The model under review builds one solid part; all positions refer to its coordinate system, in mm. Face numbers are marked on the shaded views. A direction names the side the tool comes from. Round coordinates to 2 decimals unless told otherwise and drop trailing zeros. Write each loop counter-clockwise with the first axis right and the second up, starting at its lowest first coordinate (ties: lowest second). Pieces come first, ordered by that corner, then holes. Notation, with made-up numbers: (-11, 86) -> (33, 86) arc R22 cw to (33, 101) -> close; hole circle Ø10 at (52.5, 86.5). An arc over 180 degrees is marked (long way). Return JSON: item names as keys, results as strings. Group by question number.
1. Tool access review of the marked faces 5, 6 and 7: name each direction out of +Z, -Z, +X, -X, +Y, -Y from which nothing blocks a thin tool from reaching the whole face with its end or side.
2. Take a section at A-A, the plane x = -60. Write out the cut boundary in (y, z).
3. Clearance check with flat-ended pins moving along their axes: P1, Ø4, axis at x = -89.5, z = 44, coming from the +Y side; P2, Ø4, axis at y = -20, z = -13.5, coming from the +X side; P3, Ø8, axis at x = -8.5, y = -31.5, coming from the +Z side; P4, Ø5.5, axis at x = -83.5, y = -37, coming from the +Z side. State where each tip first meets the part, or that it passes through.
4. Take a section at D-D, the plane x = -89. Write out the cut boundary in (y, z), then the cut area to 3 significant figures.
5. Mouldability with a two-part tool opening along Z and no side actions: class the marked faces 1, 2, 3 and 4 as pulls with the +Z half, pulls with the -Z half, needs draft (parallel to the pull), parting line crosses it, or undercut.
6. Take a section at B-B, the plane y = -3.5. Write out the cut boundary in (x, z), then the cut area to 3 significant figures.
7. Take a section at C-C, the plane z = 23. Write out the cut boundary in (x, y), then the cut area to 3 significant figures.
8. For line 1 along Y through (x, z) = (-63.5, 57.5) (3 decimals); line 2 along Z through (x, y) = (-63.5, -47); line 3 along X through (y, z) = (-44, -16), list the stretches that pass through material, from the lowest coordinate up. Write a range as from..to.
from build123d import *

# Parameters (mm, degrees)
F1_DEPTH = 127
F3_DEPTH = 57.15
F4_R     = 12.7
F5_DEPTH = 44.45
F6_R     = 5.08
F7_DEPTH = 13.7612578348


with BuildPart() as f1:
    # F0 (on Right) → F1 (new body)
    with BuildSketch(Plane.YZ):
        Polygon((-57.15, 0), (0, 0), (0, 63.5), (-12.7, 63.5), (-12.7, 12.7), (-57.15, 12.7), align=None)
    extrude(amount=-F1_DEPTH)

    # F2 (on face) → F3 (join)
    with BuildSketch(Plane.XZ.offset(57.15)):
        Polygon((-50.8, 0), (-63.5, 0), (-76.2, 0), (-76.2, -8.89), (-95.25, -8.89), (-95.25, -21.59), (-31.75, -21.59), (-31.75, -8.89), (-50.8, -8.89), align=None)
    extrude(amount=-F3_DEPTH)

    # F4 (on face) → F5 (join, through all)
    with BuildSketch(Plane.XZ.offset(12.7)):
        with BuildLine():
            Line((-111.125, 12.7), (-15.875, 12.7))
            Line((-15.875, 12.7), (-42.4065743945, 52.2501730104))
            ThreePointArc((-42.4065743945, 52.2501730104), (-63.5, 63.5), (-84.5934256055, 52.2501730104))
            Line((-84.5934256055, 52.2501730104), (-111.125, 12.7))
        make_face()
        with Locations((-63.5, 38.1)):
            Circle(F4_R, mode=Mode.SUBTRACT)
    extrude(amount=F5_DEPTH)

    # F6 (on face) → F7 (cut, through all)
    with BuildSketch(Plane.XY.offset(63.5)):
        with Locations((-63.5, -34.925)):
            Circle(F6_R)
    extrude(amount=-F7_DEPTH, mode=Mode.SUBTRACT)


solid = f1.part
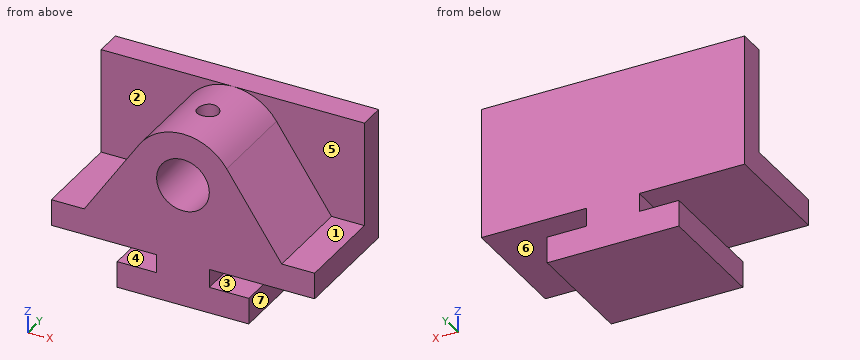
Output:
{
 "1": {"face 5": "+Z, +X, -Y", "face 6": "+X, +Y, -Y", "face 7": "-Z, +X, +Y, -Y"},
 "2": {"outline": "(-57.15, -21.59) -> (0, -21.59) -> (0, 63.5) -> (-12.7, 63.5) -> (-12.7, 63.26) -> (-31.24, 63.26) -> (-31.24, 50.31) -> (-12.7, 50.31) -> (-12.7, 25.89) -> (-57.15, 25.89) -> close; (-57.15, 50.31) -> (-38.61, 50.31) -> (-38.61, 63.26) -> (-57.15, 63.26) -> close"},
 "3": {"P1": "stops at y = 0", "P2": "stops at x = -31.75", "P3": "stops at z = 12.7", "P4": "stops at z = 56.74"},
 "4": {"outline": "(-57.15, -21.59) -> (0, -21.59) -> (0, -8.89) -> (-57.15, -8.89) -> close; (-57.15, 0) -> (0, 0) -> (0, 63.5) -> (-12.7, 63.5) -> (-12.7, 45.68) -> (-57.15, 45.68) -> close", "area": "3,560 mm^2"},
 "5": {"face 1": "pulls with the +Z half", "face 2": "needs draft", "face 3": "undercut", "face 4": "undercut"},
 "6": {"outline": "(-127, 0) -> (-76.2, 0) -> (-76.2, -8.89) -> (-95.25, -8.89) -> (-95.25, -21.59) -> (-31.75, -21.59) -> (-31.75, -8.89) -> (-50.8, -8.89) -> (-50.8, 0) -> (0, 0) -> (0, 63.5) -> (-127, 63.5) -> close", "area": "9,100 mm^2"},
 "7": {"outline": "(-127, -12.7) -> (-104.22, -12.7) -> (-104.22, -57.15) -> (-22.78, -57.15) -> (-22.78, -12.7) -> (0, -12.7) -> (0, 0) -> (-127, 0) -> close", "area": "5,230 mm^2"},
 "8": {"line 1": "y = -57.15..-40.005, -29.845..0", "line 2": "z = -21.59..25.4, 50.8..63.5", "line 3": "x = -95.25..-31.75"}
}
